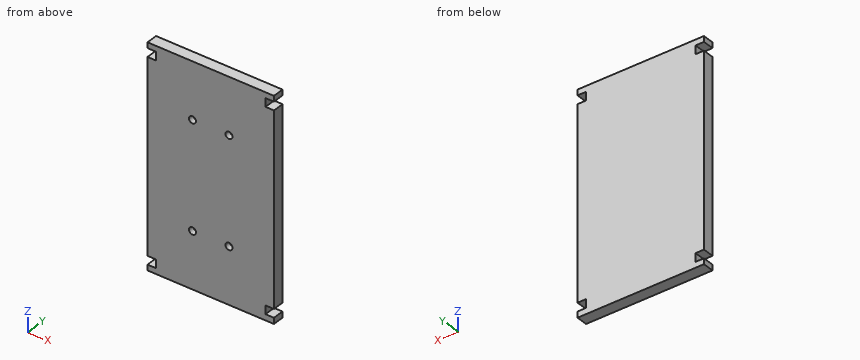
from build123d import *

# Parameters (mm, degrees)
F0_W      = 71.4375
F0_H      = 123.825
F1_DEPTH  = 6.35
F2_W      = 6.35
F2_H      = 4.7625
F3_DEPTH  = 4.7625
F4_W      = 6.35
F4_H      = 4.7625
F5_DEPTH  = 4.7625
F6_W      = 6.35
F6_H      = 4.7625
F7_DEPTH  = 4.7625
F8_W      = 6.35
F8_H      = 4.7625
F9_DEPTH  = 4.7625
F10_R     = 1.984375
F11_DEPTH = 3.175


with BuildPart() as f1:
    # F0 (on Front) → F1 (new body)
    with BuildSketch(Plane.XZ):
        with Locations((1.604452, 25.450979)):
            Rectangle(F0_W, F0_H)
    extrude(amount=F1_DEPTH)

    # F2 (on face) → F3 (cut)
    with BuildSketch(Plane.YZ.offset(37.323202)):
        with Locations((-3.175, 81.807229)):
            Rectangle(F2_W, F2_H)
    extrude(amount=-F3_DEPTH, mode=Mode.SUBTRACT)

    # F4 (on face) → F5 (cut)
    with BuildSketch(Plane.YZ.offset(37.323202)):
        with Locations((-3.175, -30.70041)):
            Rectangle(F4_W, F4_H)
    extrude(amount=-F5_DEPTH, mode=Mode.SUBTRACT)

    # F6 (on face) → F7 (cut)
    with BuildSketch(Plane(origin=(-34.114298, 0, 0), x_dir=(0, -1, 0), z_dir=(-1, 0, 0))):
        with Locations((3.175, 81.807229)):
            Rectangle(F6_W, F6_H)
    extrude(amount=-F7_DEPTH, mode=Mode.SUBTRACT)

    # F8 (on face) → F9 (cut)
    with BuildSketch(Plane(origin=(-34.114298, 0, 0), x_dir=(0, -1, 0), z_dir=(-1, 0, 0))):
        with Locations((3.175, -30.905271)):
            Rectangle(F8_W, F8_H)
    extrude(amount=-F9_DEPTH, mode=Mode.SUBTRACT)

    # F10 (on face) → F11 (cut)
    with BuildSketch(Plane.XZ.offset(6.35)):
        with Locations((-8.714298, 55.613479)):
            Circle(F10_R)
        with Locations((11.923202, 55.613479)):
            Circle(F10_R)
        with Locations((-8.714298, -4.711521)):
            Circle(F10_R)
        with Locations((11.923202, -4.711521)):
            Circle(F10_R)
    extrude(amount=-F11_DEPTH, mode=Mode.SUBTRACT)


solid = f1.part
Read the model definition and answer for the solid it produces. Units are mm, in the model's axes. Round coordinates to 2 decimals unless told otherwise and drop trailing zeros. Order: outer loops, then holes, each group sorted by start corner. A loop starts at its lowest first (then second) coordinate and runs counter-clockwise, first axis right, second up.
1) The part is cut by section A-A on y = -5. Write down the section's boundary in (x, z), plus the area to 3 significant figures.
2) Straight lines are drawn through the part: L1, parallel to Z at x = -30, y = -5.5; L2, parallel to X at y = -3.5, z = -6. For each, find the intervals that lie inside material, in ascending order.
3) Flat-ended cylindrical pins translate along their axes: pin 1 (1.4 mm diameter, centred on y = -2, z = -31, fed in from -X); pin 2 (3 mm diameter, centred on x = -8, z = 55.5, fed in from -Y); pin 3 (3 mm diameter, centred on x = -8.71, z = -4.71, fed in from -Y) (3 decimals). Find the tip coordinate at first contact, or state that the pin passes through.
Resolved:
1. outline: (-34.11, -36.46) - (37.32, -36.46) - (37.32, -33.08) - (32.56, -33.08) - (32.56, -28.32) - (37.32, -28.32) - (37.32, 79.43) - (32.56, 79.43) - (32.56, 84.19) - (37.32, 84.19) - (37.32, 87.36) - (-34.11, 87.36) - (-34.11, 84.19) - (-29.35, 84.19) - (-29.35, 79.43) - (-34.11, 79.43) - (-34.11, -28.52) - (-29.35, -28.52) - (-29.35, -33.29) - (-34.11, -33.29) - close; hole circle Ø3.97 at (-8.71, -4.71); hole circle Ø3.97 at (-8.71, 55.61); hole circle Ø3.97 at (11.92, -4.71); hole circle Ø3.97 at (11.92, 55.61)
1. area: 8,710 mm2
2. L1: z = -36.46 to -33.29, -28.52 to 79.43, 84.19 to 87.36
2. L2: x = -34.11 to -10.22, -7.21 to 10.41, 13.43 to 37.32
3. pin 1: stops at x = -29.35
3. pin 2: stops at y = -6.35
3. pin 3: stops at y = -3.175
